Here's how the part is built. I have some questions about the finished solid (model axes, mm). A direction names the side the tool comes from. Coordinates: 2 decimals unless noted, no trailing zeros. Order: outer loops, then holes, each group sorted by start corner. A loop starts at its lowest first (then second) coordinate and runs counter-clockwise, first axis right, second up. Notation, with made-up numbers: (73.25, -27) - (118.25, -27) arc R32 ccw to (118.25, 12) - close; hole circle Ø1 at (10.5, 61.5). An arc over 180 degrees is marked (long way). Answer as CSV lines item,"result". Start each with the question number.
Item 1: On a 3-axis mill with a long thin cutter (end or side, diameter ignored), from which of +Z, -Z, +X, -X, +Y, -Y can I reach the whole of each face in a straight line? I mean faces 1 (the face through (0, 1, 26.93)), 2 (the face through (0, 1, 18.361)). Say none if no direction works.
Item 2: Imagine slicing it at B-B on x = 8. List the corners of the cut face in (y, z) for me, and give its area (3 significant figures).
Item 3: I'm going to push a flat-ended pin straight in: pin 1 (1 mm diameter, centred on x = -2, z = -13, fed in from -Y). Where does the tip first touch, or does it pass through?
Item 4: We'd pull the mould along Z, two halves only. Please class faces 3 (the face through (0, 0, 0)), 4 (the face through (0, 1, -26.93)), 5 (the face through (14.75, 0.79, 19.64)): pulls with the +Z half, pulls with the -Z half, needs draft (parallel to the pull), parting line crosses it, or undercut.
Item 5: I need wall thicknesses on line 1 (Z direction, x = 11.5, y = 0.2); line 2 (Z direction, x = -14, y = 1.3). Which ranges of each line are inside material? Lowest first, please.
Item 6: Imagine slicing it at A-A on y = 1.2. List the corners of the cut face in (x, z) for me.
from build123d import *

# Parameters (mm, degrees)
SKIZZE1_W                       = 41.517188714
SKIZZE1_H                       = 53.860351018
AUFSATZ_LINEAR_AUSTRAGEN1_DEPTH = 1.6


with BuildPart() as part:
    # Skizze1 → Aufsatz-Linear austragen1 (new body)
    with BuildSketch(Plane(origin=(0, 0, 0), x_dir=(1, 0, 0), z_dir=(0, 1, 0))):
        Rectangle(SKIZZE1_W, SKIZZE1_H)
        with BuildLine():
            ThreePointArc((-13.5, -18.360991054), (-14.75, -19.610991054), (-13.5, -20.860991054))
            Line((-13.5, -20.860991054), (13.5, -20.860991054))
            ThreePointArc((13.5, -20.860991054), (14.75, -19.610991054), (13.5, -18.360991054))
            Line((13.5, -18.360991054), (-13.5, -18.360991054))
        make_face(mode=Mode.SUBTRACT)
    extrude(amount=AUFSATZ_LINEAR_AUSTRAGEN1_DEPTH)


solid = part.part
Responses:
1,face 1,"+Z, +X, -X, +Y, -Y"
1,face 2,"+Y, -Y"
2,outline,"(0, -26.93) - (1.6, -26.93) - (1.6, 18.36) - (0, 18.36) - close; (0, 20.86) - (1.6, 20.86) - (1.6, 26.93) - (0, 26.93) - close"
2,area,"82.2 mm^2"
3,pin 1,"stops at y = 0"
4,face 3,"needs draft"
4,face 4,"pulls with the -Z half"
4,face 5,"undercut"
5,line 1,"z = -26.93 to 18.36, 20.86 to 26.93"
5,line 2,"z = -26.93 to 18.47, 20.76 to 26.93"
6,outline,"(-20.76, -26.93) - (20.76, -26.93) - (20.76, 26.93) - (-20.76, 26.93) - close; hole (-13.5, 18.36) - (13.5, 18.36) arc R1.25 ccw to (13.5, 20.86) - (-13.5, 20.86) arc R1.25 ccw to start"
